```python
from build123d import *

# Parameters (mm, degrees)
SKIZZE1_W                       = 8
SKIZZE1_H                       = 11.8
AUFSATZ_LINEAR_AUSTRAGEN1_DEPTH = 2.5
SKIZZE2_W                       = 8
SKIZZE2_H                       = 1.5
AUFSATZ_LINEAR_AUSTRAGEN2_DEPTH = 1.3
SKIZZE3_W                       = 2.2
SKIZZE3_H                       = 1.5
AUFSATZ_LINEAR_AUSTRAGEN3_DEPTH = 1.2
AUFSATZ_LINEAR_AUSTRAGEN4_DEPTH = 1.75
AUFSATZ_LINEAR_AUSTRAGEN5_DEPTH = 0.05
SKIZZE6_W                       = 2
SKIZZE6_H                       = 3.5
SCHNITT_LINEAR_AUSTRAGEN1_DEPTH = 11.3
SKIZZE7_W                       = 2
SKIZZE7_H                       = 4.5
SCHNITT_LINEAR_AUSTRAGEN2_DEPTH = 1
SKIZZE8_W                       = 1
SKIZZE8_H                       = 1
SCHNITT_LINEAR_AUSTRAGEN3_DEPTH = 13.574975149
FASE1_SIZE                      = 0.4
LINEARES_MUSTER1_COUNT          = 3
LINEARES_MUSTER1_PITCH          = 2.5
FASE1_OF_LINEARES_MUSTER1_SIZE  = 0.4
AUFSATZ_LINEAR_AUSTRAGEN6_DEPTH = 2
SCHNITT_LINEAR_AUSTRAGEN4_DEPTH = 2.5
LINEARES_MUSTER2_COUNT          = 7
LINEARES_MUSTER2_PITCH          = 0.5
VERRUNDUNG1_R                   = 2
VERRUNDUNG2_R                   = 0.2
SPIEGELN1_COPY_1_DEPTH          = 2.5
SPIEGELN1_COPY_2_DEPTH          = 2.5
SPIEGELN1_COPY_3_DEPTH          = 2.5
SPIEGELN1_COPY_4_DEPTH          = 2.5
SPIEGELN1_COPY_5_DEPTH          = 2.5
SPIEGELN1_COPY_6_DEPTH          = 2.5
VERRUNDUNG1_OF_SPIEGELN1_R      = 2
VERRUNDUNG2_OF_SPIEGELN1_R      = 0.2


with BuildPart() as part:
    # Skizze1 → Aufsatz-Linear austragen1 (new, symmetric)
    with BuildSketch(Plane.XY):
        with Locations((0, 5.9)):
            Rectangle(SKIZZE1_W, SKIZZE1_H)
    extrude(amount=AUFSATZ_LINEAR_AUSTRAGEN1_DEPTH, both=True)

    # Skizze2 → Aufsatz-Linear austragen2 (add)
    with BuildSketch(Plane.XY.offset(2.5)):
        with Locations((0, 0.75)):
            Rectangle(SKIZZE2_W, SKIZZE2_H)
    extrude(amount=AUFSATZ_LINEAR_AUSTRAGEN2_DEPTH)

    # Skizze3 → Aufsatz-Linear austragen3 (add)
    with BuildSketch(Plane(origin=(0, 0, -2.5), x_dir=(-1, 0, 0), z_dir=(0, 0, -1))):
        with Locations((-2.9, 0.75)):
            Rectangle(SKIZZE3_W, SKIZZE3_H)
        with Locations((2.9, 0.75)):
            Rectangle(SKIZZE3_W, SKIZZE3_H)
    extrude(amount=AUFSATZ_LINEAR_AUSTRAGEN3_DEPTH)

    # Skizze4 → Aufsatz-Linear austragen4 (add, symmetric)
    with BuildSketch(Plane(origin=(0, 0, 0), x_dir=(0, 0, -1), z_dir=(1, 0, 0))):
        Polygon((2.5, 11.8), (3.5, 10.9), (3.5, 10.4), (2.5, 10.4), align=None)
    extrude(amount=AUFSATZ_LINEAR_AUSTRAGEN4_DEPTH, both=True)

    # Skizze5 → Aufsatz-Linear austragen5 (add)
    with BuildSketch(Plane(origin=(0, 0, -2.5), x_dir=(-1, 0, 0), z_dir=(0, 0, -1))):
        Polygon((1.8, 1.5), (2.9, 2.8), (4, 1.5), align=None)
    extrude(amount=AUFSATZ_LINEAR_AUSTRAGEN5_DEPTH)

    # Skizze6 → Schnitt-Linear austragen1 (cut)
    with BuildSketch(Plane.XZ):
        with Locations((-2.5, -0.25)):
            Rectangle(SKIZZE6_W, SKIZZE6_H)
    schnitt_linear_austragen1 = extrude(amount=-SCHNITT_LINEAR_AUSTRAGEN1_DEPTH, mode=Mode.SUBTRACT)

    # Skizze7 → Schnitt-Linear austragen2 (cut)
    with BuildSketch(Plane.XY.offset(2.5)):
        with Locations((-2.5, 9.55)):
            Rectangle(SKIZZE7_W, SKIZZE7_H)
    schnitt_linear_austragen2 = extrude(amount=-SCHNITT_LINEAR_AUSTRAGEN2_DEPTH, mode=Mode.SUBTRACT)

    # Skizze8 → Schnitt-Linear austragen3 (cut, through all)
    with BuildSketch(Plane.XZ.offset(-11.3)):
        with Locations((-2.5, -1)):
            Rectangle(SKIZZE8_W, SKIZZE8_H)
    schnitt_linear_austragen3 = extrude(amount=-SCHNITT_LINEAR_AUSTRAGEN3_DEPTH, mode=Mode.SUBTRACT)

    # Fase1
    fase1_edges = [part.edges().sort_by_distance(p)[0] for p in [
        (-3, 11.8, -1),
        (-2.5, 11.8, -0.5),
        (-2, 11.8, -1),
        (-2.5, 11.8, -1.5),
    ]]
    chamfer(fase1_edges, length=FASE1_SIZE)

    # Lineares Muster1: Schnitt-Linear austragen1, Schnitt-Linear austragen2, Schnitt-Linear austragen3 ×3
    with Locations(*[(i * LINEARES_MUSTER1_PITCH, 0, 0) for i in range(1, LINEARES_MUSTER1_COUNT)]):
        add(schnitt_linear_austragen1, mode=Mode.SUBTRACT)
        add(schnitt_linear_austragen2, mode=Mode.SUBTRACT)
        add(schnitt_linear_austragen3, mode=Mode.SUBTRACT)

    # Fase1 of Lineares Muster1
    fase1_of_lineares_muster1_edges = [part.edges().sort_by_distance(p)[0] for p in [
        (-0.5, 11.8, -1),
        (0, 11.8, -0.5),
        (0.5, 11.8, -1),
        (0, 11.8, -1.5),
        (2, 11.8, -1),
        (2.5, 11.8, -0.5),
        (3, 11.8, -1),
        (2.5, 11.8, -1.5),
    ]]
    chamfer(fase1_of_lineares_muster1_edges, length=FASE1_OF_LINEARES_MUSTER1_SIZE)

    # Skizze9 → Aufsatz-Linear austragen6 (add, symmetric)
    with BuildSketch(Plane.XY):
        Polygon((-4, 7.8), (-7, 4.8), (-5.6, 0.8), (-5.5, 0.8), (-5.5, 4.885786438), (-4, 6.385786438), align=None)
    aufsatz_linear_austragen6 = extrude(amount=AUFSATZ_LINEAR_AUSTRAGEN6_DEPTH, both=True)

    # Skizze11 → Schnitt-Linear austragen4 (cut, symmetric)
    with BuildSketch(Plane.XY):
        Polygon((-5.940175212, 1.771929178), (-5.775, 1.771929178), (-5.775, 1.3), align=None)
    schnitt_linear_austragen4 = extrude(amount=SCHNITT_LINEAR_AUSTRAGEN4_DEPTH, both=True, mode=Mode.SUBTRACT)

    # Lineares Muster2: Schnitt-Linear austragen4 ×7
    with Locations(*[Vector(-0.33035042472810877, 0.9438583563660166, 0) * (i * LINEARES_MUSTER2_PITCH) for i in range(1, LINEARES_MUSTER2_COUNT)]):
        add(schnitt_linear_austragen4, mode=Mode.SUBTRACT)

    # Verrundung1
    verrundung1_edges = [part.edges().sort_by_distance(p)[0] for p in [
        (-5.5, 4.885786438, 0),
    ]]
    fillet(verrundung1_edges, radius=VERRUNDUNG1_R)

    # Verrundung2
    verrundung2_edges = [part.edges().sort_by_distance(p)[0] for p in [
        (-4, 6.385786438, 0),
    ]]
    fillet(verrundung2_edges, radius=VERRUNDUNG2_R)

    # Spiegeln1: Aufsatz-Linear austragen6, Schnitt-Linear austragen4 across plane
    add(aufsatz_linear_austragen6.mirror(Plane(origin=(0, 0, 0), x_dir=(0, 0, 1), z_dir=(1, 0, 0))))
    add(schnitt_linear_austragen4.mirror(Plane(origin=(0, 0, 0), x_dir=(0, 0, 1), z_dir=(1, 0, 0))), mode=Mode.SUBTRACT)

    # Spiegeln1 copy 1 sketch → Spiegeln1 copy 1 (cut, symmetric)
    with BuildSketch(Plane(origin=(0.165175212, 0.471929178, 0), x_dir=(-1, 0, 0), z_dir=(0, 0, 1))):
        Polygon((-5.940175212, -1.771929178), (-5.775, -1.771929178), (-5.775, -1.3), align=None)
    extrude(amount=SPIEGELN1_COPY_1_DEPTH, both=True, mode=Mode.SUBTRACT)

    # Spiegeln1 copy 2 sketch → Spiegeln1 copy 2 (cut, symmetric)
    with BuildSketch(Plane(origin=(0.33035042472810877, 0.9438583563660166, 0), x_dir=(-1, 0, 0), z_dir=(0, 0, 1))):
        Polygon((-5.940175212, -1.771929178), (-5.775, -1.771929178), (-5.775, -1.3), align=None)
    extrude(amount=SPIEGELN1_COPY_2_DEPTH, both=True, mode=Mode.SUBTRACT)

    # Spiegeln1 copy 3 sketch → Spiegeln1 copy 3 (cut, symmetric)
    with BuildSketch(Plane(origin=(0.495525637, 1.415787535, 0), x_dir=(-1, 0, 0), z_dir=(0, 0, 1))):
        Polygon((-5.940175212, -1.771929178), (-5.775, -1.771929178), (-5.775, -1.3), align=None)
    extrude(amount=SPIEGELN1_COPY_3_DEPTH, both=True, mode=Mode.SUBTRACT)

    # Spiegeln1 copy 4 sketch → Spiegeln1 copy 4 (cut, symmetric)
    with BuildSketch(Plane(origin=(0.660700849, 1.887716713, 0), x_dir=(-1, 0, 0), z_dir=(0, 0, 1))):
        Polygon((-5.940175212, -1.771929178), (-5.775, -1.771929178), (-5.775, -1.3), align=None)
    extrude(amount=SPIEGELN1_COPY_4_DEPTH, both=True, mode=Mode.SUBTRACT)

    # Spiegeln1 copy 5 sketch → Spiegeln1 copy 5 (cut, symmetric)
    with BuildSketch(Plane(origin=(0.825876062, 2.359645891, 0), x_dir=(-1, 0, 0), z_dir=(0, 0, 1))):
        Polygon((-5.940175212, -1.771929178), (-5.775, -1.771929178), (-5.775, -1.3), align=None)
    extrude(amount=SPIEGELN1_COPY_5_DEPTH, both=True, mode=Mode.SUBTRACT)

    # Spiegeln1 copy 6 sketch → Spiegeln1 copy 6 (cut, symmetric)
    with BuildSketch(Plane(origin=(0.991051274, 2.831575069, 0), x_dir=(-1, 0, 0), z_dir=(0, 0, 1))):
        Polygon((-5.940175212, -1.771929178), (-5.775, -1.771929178), (-5.775, -1.3), align=None)
    extrude(amount=SPIEGELN1_COPY_6_DEPTH, both=True, mode=Mode.SUBTRACT)

    # Verrundung1 of Spiegeln1
    verrundung1_of_spiegeln1_edges = [part.edges().sort_by_distance(p)[0] for p in [
        (5.5, 4.885786438, 0),
    ]]
    fillet(verrundung1_of_spiegeln1_edges, radius=VERRUNDUNG1_OF_SPIEGELN1_R)

    # Verrundung2 of Spiegeln1
    verrundung2_of_spiegeln1_edges = [part.edges().sort_by_distance(p)[0] for p in [
        (4, 6.385786438, 0),
    ]]
    fillet(verrundung2_of_spiegeln1_edges, radius=VERRUNDUNG2_OF_SPIEGELN1_R)


solid = part.part
```
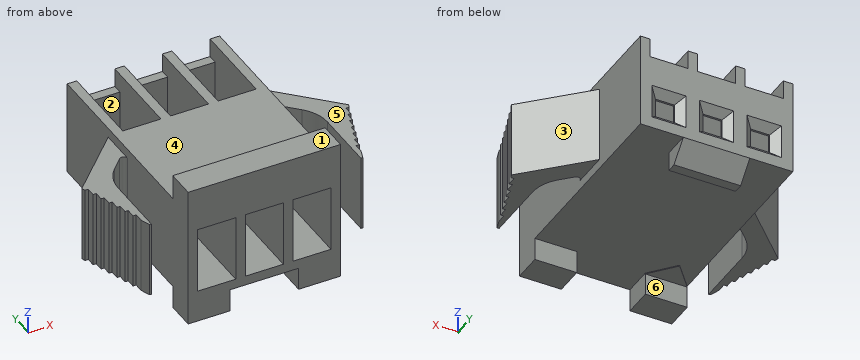
Can you work these out from the model? Positions are in its coordinate system, mm. Face numbers are marked on the shaded views. A direction names the side the tool comes from. Round coordinates to 2 decimals unless told otherwise and drop trailing zeros. Loops run counter-clockwise (first coordinate to the right, second up) from the corner with the lowest first, then second, coordinate; pieces in that order, holes last. Notation, with made-up numbers: (41.5, -38) -> (85.5, -38) arc R25 cw to (85.5, -7) -> close; hole circle Ø1 at (83, -24). An arc over 180 degrees is marked (long way). Answer in a Markdown table with one row per item.
Item 1: Suppose I cut it at C-C, the plane y = 8.75. List the corners of the cut face in (x, z) for me.
Answer block:
| item | result |
|---|---|
| outline | (-4, -2.5) -> (4, -2.5) -> (4, 2.5) -> (3.5, 2.5) -> (3.5, -2) -> (1.5, -2) -> (1.5, 2.5) -> (1, 2.5) -> (1, -2) -> (-1, -2) -> (-1, 2.5) -> (-1.5, 2.5) -> (-1.5, -2) -> (-3.5, -2) -> (-3.5, 2.5) -> (-4, 2.5) -> close |
Item 2: If I drill on probe 1 along X at (y, z) = (2.75, -0.5); probe 2 along X at (y, z) = (10.25, -1.25); probe 3 along X at (y, z) = (2, -1.75), over which ranges is the centre line in solid material (lowest first)?
Answer block:
| item | result |
|---|---|
| probe 1 | -6.27 to -5.5, -4 to -3.5, -1.5 to -1, 1 to 1.5, 3.5 to 4, 5.5 to 6.27 |
| probe 2 | -4 to -3.5, -1.5 to -1, 1 to 1.5, 3.5 to 4 |
| probe 3 | -5.94 to -5.5, -4 to -3.5, -1.5 to -1, 1 to 1.5, 3.5 to 4, 5.5 to 5.94 |
Item 3: We'd pull the mould along X, two halves only. Please class the marked faces 1, 2 and 3: released by +X, released by -X, zero draft, split by the parting line, or undercut.
Answer block:
| item | result |
|---|---|
| face 1 | zero draft |
| face 2 | undercut |
| face 3 | released by +X |
Item 4: Will these pins go through, and if not, where does the flat tip stop? P1, Ø1.6, axis at x = -2, y = 6, coming from the +Z side; P2, Ø4, axis at y = 5, z = 0, coming from the -X side; P3, Ø3, axis at y = 10, z = 2, coming from the -X side; P4, Ø3, axis at x = -2, z = -2.5, coming from the -Y side.
Answer block:
| item | result |
|---|---|
| P1 | z = 2.5 |
| P2 | x = -7 |
| P3 | x = -4 |
| P4 | y = 0 |
Item 5: Suppose I cut it at D-D, the plane z = -2.75. List the corners of the cut face in (x, y) for me (3 decimals), plus the area to 3 significant figures.
Answer block:
| item | result |
|---|---|
| outline | (-4, 0) -> (-1.8, 0) -> (-1.8, 1.5) -> (-4, 1.5) -> close; (-1.75, 10.4) -> (1.75, 10.4) -> (1.75, 11.575) -> (-1.75, 11.575) -> close; (1.8, 0) -> (4, 0) -> (4, 1.5) -> (1.8, 1.5) -> close |
| area | 10.7 mm² |
Item 6: Suppose I cut it at A-A, the plane y = 3.5. List the corners of the cut face in (x, z) for me.
Answer block:
| item | result |
|---|---|
| outline | (-6.44, -2) -> (-5.5, -2) -> (-5.5, 2) -> (-6.44, 2) -> close; (-4, -2.5) -> (4, -2.5) -> (4, 2.5) -> (-4, 2.5) -> close; (5.5, -2) -> (6.44, -2) -> (6.44, 2) -> (5.5, 2) -> close; hole (-3.5, -2) -> (-1.5, -2) -> (-1.5, 1.5) -> (-3.5, 1.5) -> close; hole (-1, -2) -> (1, -2) -> (1, 1.5) -> (-1, 1.5) -> close; hole (1.5, -2) -> (3.5, -2) -> (3.5, 1.5) -> (1.5, 1.5) -> close |
Item 7: On a 3-axis mill with a long thin cutter (end or side, diameter ignored), from which of +Z, -Z, +X, -X, +Y, -Y can I reach the whole of each face in a straight line? I mean the marked faces 4, 5 and 6. Say none if no direction works.
Answer block:
| item | result |
|---|---|
| face 4 | +Z, +X, -X, +Y |
| face 5 | +Z, +X, +Y, -Y |
| face 6 | -Z, +X, -X, +Y |
Item 8: Suppose I cut it at B-B, the plane x = 2.5. List the corners of the cut face in (y, z) for me, plus the area to 3 significant figures.
Answer block:
| item | result |
|---|---|
| outline | (0, -3.7) -> (1.5, -3.7) -> (1.5, -2.5) -> (11.8, -2.5) -> (11.8, -1.9) -> (11.4, -1.5) -> (11.3, -1.5) -> (11.3, -2) -> (0, -2) -> close; (0, 1.5) -> (7.3, 1.5) -> (7.3, 2.5) -> (1.5, 2.5) -> (1.5, 3.8) -> (0, 3.8) -> close; (11.3, -0.5) -> (11.4, -0.5) -> (11.8, -0.1) -> (11.8, 1.5) -> (11.3, 1.5) -> close |
| area | 18.0 mm² |
